from build123d import *

# Parameters (mm, degrees)
SALIENTE_EXTRUIR1_DEPTH = 12
SALIENTE_EXTRUIR2_DEPTH = 2.5
REDONDEO2_R             = 0.5
SALIENTE_EXTRUIR4_DEPTH = 14.5
REDONDEO5_R             = 1


with BuildPart() as part:
    # Croquis1 → Saliente-Extruir1 (new body)
    with BuildSketch(Plane(origin=(0, 0, 0), x_dir=(1, 0, 0), z_dir=(0, 1, 0))):
        Polygon((8.544783984006465, -6.5e-16), (4.272391992003232, 7.400000000000002), (-4.27239199200323, 7.400000000000003), (-8.544783984006463, 1.3e-15), (-4.272391992003225, -7.400000000000005), (4.272391992003232, -7.400000000000004), align=None)
        Polygon((-3.6950417228136043, 6.400000000000002), (-7.390083445627212, 8.7e-16), (-3.6950417228136003, -6.400000000000005), (3.695041722813607, -6.400000000000004), (7.390083445627214, -1.74e-15), (3.695041722813606, 6.400000000000002), align=None, mode=Mode.SUBTRACT)
    extrude(amount=SALIENTE_EXTRUIR1_DEPTH)

    # Croquis2 → Saliente-Extruir2 (add)
    with BuildSketch(Plane.XZ):
        Polygon((8.544783984006465, 6.5e-16), (4.272391992003232, 7.400000000000004), (-4.272391992003225, 7.400000000000005), (-8.544783984006463, -1.3e-15), (-4.27239199200323, -7.400000000000003), (4.272391992003232, -7.400000000000002), align=None)
    extrude(amount=SALIENTE_EXTRUIR2_DEPTH)

    # Redondeo2
    redondeo2_edges = [part.edges().sort_by_distance(p)[0] for p in [
        (8.9e-16, 12, -6.400000000000002),
        (-5.542562584220408, 12, -3.2000000000000015),
        (-5.5425625842204065, 12, 3.200000000000002),
        (3.11e-15, 12, 6.400000000000005),
        (5.542562584220411, 12, 3.200000000000003),
        (5.54256258422041, 12, -3.2),
    ]]
    fillet(redondeo2_edges, radius=REDONDEO2_R)

    # Croquis3 → Saliente-Extruir4 (add)
    with BuildSketch(Plane.XZ.offset(2.5)):
        with BuildLine():
            Line((4.272391992003232, 7.400000000000004), (8.544783984006465, 6.5e-16))
            ThreePointArc((8.544783984006463, 0), (7.400000000000001, 4.272391992003231), (4.2723919920032305, 7.400000000000002))
        make_face()
        with BuildLine():
            ThreePointArc((4.2723919920032305, 7.400000000000002), (2.42e-15, 8.544783984006463), (-4.272391992003226, 7.400000000000004))
            Line((-4.272391992003225, 7.400000000000005), (4.272391992003232, 7.400000000000004))
        make_face()
        with BuildLine():
            ThreePointArc((-4.272391992003226, 7.400000000000004), (-7.3999999999999995, 4.272391992003234), (-8.544783984006463, 1.05e-15))
            Line((-8.544783984006463, -8.9e-16), (-4.272391992003225, 7.400000000000005))
        make_face()
        with BuildLine():
            ThreePointArc((-8.544783984006463, 1.05e-15), (-7.400000000000001, -4.272391992003232), (-4.272391992003228, -7.400000000000003))
            Line((-4.27239199200323, -7.400000000000003), (-8.544783984006463, -1.3e-15))
        make_face()
        with BuildLine():
            Line((4.272391992003231, -7.400000000000002), (-4.27239199200323, -7.400000000000003))
            ThreePointArc((-4.272391992003228, -7.400000000000003), (-1.57e-15, -8.544783984006463), (4.272391992003226, -7.400000000000005))
        make_face()
        with BuildLine():
            Line((8.544783984006465, 8.9e-16), (4.272391992003232, -7.400000000000002))
            ThreePointArc((4.272391992003226, -7.400000000000005), (7.399999999999999, -4.272391992003235), (8.544783984006463, -2.09e-15))
        make_face()
    extrude(amount=-SALIENTE_EXTRUIR4_DEPTH)

    # Redondeo5
    redondeo5_edges = [part.edges().sort_by_distance(p)[0] for p in [
        (8.544783984006457, -2.5, -2.9e-16),
    ]]
    fillet(redondeo5_edges, radius=REDONDEO5_R)


solid = part.part
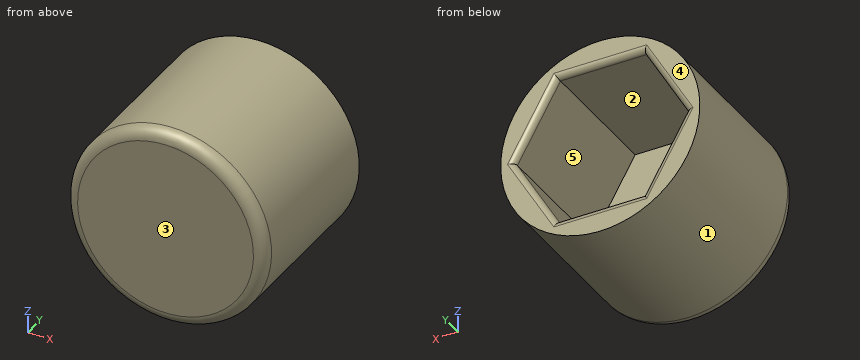
Input: part model. Units: mm. Frame: model coordinates. Face numbers are marked on the shaded views. A direction names the side the tool comes from. Round coordinates to 2 decimals unless told otherwise and drop trailing zeros. Loops run counter-clockwise (first coordinate to the right, second up) from the corner with the lowest first, then second, coordinate; pieces in that order, holes last. Notation, with made-up numbers: (79.25, 0.25) -> (130.25, 0.25) arc R21 cw to (130.25, 39.25) -> close; hole circle Ø3 at (-23.75, -9.75). An arc over 180 degrees is marked (long way). Answer as a JSON object with one key per item and string values. Group by question number.
1) Section query A-A on y = 4.5. Output: boundary loops of the cut face in (x, z), plus the area to 3 significant figures.
2) Draft query along X for the marked faces 1, 2 and 3. Return one class per face: +X half, -X half, draft (parallel to the pull), parting line (faces both ways), or undercut.
3) Ray query, L1, parallel to Z at x = -4, y = -0.25; L2, parallel to Y at x = 5.5, z = 2.75; L3, parallel to X at y = 10.5, z = 1.75. Return the intervals inside material, ascending.
4) Pin query (flat end, axial travel): pin 1 (6.5 mm diameter, centred on x = 1.5, z = -1.5, fed in from +Y); pin 2 (5 mm diameter, centred on y = 1.5, z = -5.5, fed in from +X); pin 3 (4 mm diameter, centred on x = -6.5, y = 9.5, fed in from +Z). Return the tip coordinate at first contact, or that it passes through.
5) Section query B-B on y = -1.25. Output: boundary loops of the cut face in (x, z), plus the area to 3 significant figures.
6) Reachability of the marked faces 4 and 5 from +Z, -Z, +X, -X, +Y, -Y: full face, straight path, thin tool, end or side. Return the list, or none.
Reply:
{
 "1": {"outline": "circle Ø17.09 at (0, 0); hole (-7.39, 0) -> (-3.7, -6.4) -> (3.7, -6.4) -> (7.39, 0) -> (3.7, 6.4) -> (-3.7, 6.4) -> close", "area": "87.5 mm2"},
 "2": {"face 1": "parting line", "face 2": "undercut", "face 3": "draft"},
 "3": {"L1": "z = -7.55 to 7.55", "L2": "y = -2.5 to 0", "L3": "x = -8.36 to -6.38, 6.38 to 8.36"},
 "4": {"pin 1": "stops at y = 0", "pin 2": "stops at x = 8", "pin 3": "stops at z = 7.26"},
 "5": {"outline": "circle Ø17.09 at (0, 0)", "area": "229 mm2"},
 "6": {"face 4": "+Z, -Z, +X, -X, +Y", "face 5": "+Y"}
}
